Read the model definition and answer for the solid it produces. Units are mm, in the model's axes. Face numbers are marked on the shaded views. A direction names the side the tool comes from. Coordinates: 2 decimals unless noted, no trailing zeros. Write each loop counter-clockwise with the first axis right and the second up, starting at its lowest first coordinate (ties: lowest second). Pieces come first, ordered by that corner, then holes. Notation, with made-up numbers: (-19, 61.25) - (6, 61.25) arc R10 cw to (6, 67.25) - close; hole circle Ø10 at (85, 44). An arc over 180 degrees is marked (long way). Use a Markdown table: item, result.
from build123d import *

# Parameters (mm, degrees)
F0_R     = 38.1
F1_DEPTH = 76.2
F3_DEPTH = 175.006
F5_DEPTH = 304.8
F6_DEPTH = 430.022
F7_DEPTH = 172.72
F8_SIZE  = 12.7


with BuildPart() as f1:
    # F0 (on Top) → F1 (new body)
    with BuildSketch(Plane.XY):
        with BuildLine():
            Line((304.8000000003, 0), (-304.8000000003, 0))
            ThreePointArc((-304.8000000003, 0), (-358.6815367265, -22.3184632735), (-381, -76.1999999997))
            Line((-381, -76.1999999997), (-304.8000000003, -76.1999999997))
            ThreePointArc((-304.8000000003, -76.1999999997), (-228.6, -152.4), (-304.8000000003, -228.6000000003))
            Line((-304.8000000003, -228.6000000003), (-381, -228.6000000003))
            ThreePointArc((-381, -228.6000000003), (-358.6815367265, -282.4815367265), (-304.8000000003, -304.8))
            Line((-304.8000000003, -304.8), (304.8000000003, -304.8))
            ThreePointArc((304.8000000003, -304.8), (358.6815367267, -282.4815367264), (381.0000000003, -228.6))
            Line((381, -228.6000000003), (304.8000000003, -228.6000000003))
            ThreePointArc((304.8000000003, -228.6000000003), (228.6, -152.4), (304.8000000003, -76.1999999997))
            Line((304.8000000003, -76.1999999997), (381, -76.1999999997))
            ThreePointArc((381.0000000005, -76.2000000003), (358.6815367269, -22.3184632737), (304.8000000003, 0))
        make_face()
        with Locations((-177.8, -228.6)):
            Circle(F0_R, mode=Mode.SUBTRACT)
        with Locations((177.8, -228.6)):
            Circle(F0_R, mode=Mode.SUBTRACT)
        Polygon((-25.4, -114.8846255064), (-25.4, -48.2938652754), (25.4, -48.2938652754), (25.4, -114.8846255064), (101.6, -114.8846255064), (101.6, -165.6846255064), (25.4, -165.6846255064), (25.4, -241.8846255064), (-25.4, -241.8846255064), (-25.4, -165.6846255064), (-101.6, -165.6846255064), (-101.6, -114.8846255064), align=None, mode=Mode.SUBTRACT)
        with Locations((-177.7999999997, -76.2)):
            Circle(F0_R, mode=Mode.SUBTRACT)
        with Locations((177.8, -75.2889811993)):
            Circle(F0_R, mode=Mode.SUBTRACT)
        with Locations((-177.7999999997, -76.2)):
            Circle(F0_R)
        Polygon((25.4, -48.2938652754), (-25.4, -48.2938652754), (-25.4, -114.8846255064), (-101.6, -114.8846255064), (-101.6, -165.6846255064), (-25.4, -165.6846255064), (-25.4, -241.8846255064), (25.4, -241.8846255064), (25.4, -165.6846255064), (101.6, -165.6846255064), (101.6, -114.8846255064), (25.4, -114.8846255064), align=None)
        with Locations((177.8, -75.2889811993)):
            Circle(F0_R)
        with Locations((177.8, -228.6)):
            Circle(F0_R)
        with Locations((-177.8, -228.6)):
            Circle(F0_R)
    extrude(amount=-F1_DEPTH)

    # F2 (on Top) → F3 (join)
    with BuildSketch(Plane.XY):
        Polygon((25.4, -50.8), (-25.4, -50.8), (-25.4, -127), (-101.6, -127), (-101.6, -177.8), (-25.4, -177.8), (-25.4, -254), (25.4, -254), (25.4, -177.8), (101.6, -177.8), (101.6, -127), (25.4, -127), align=None)
    extrude(amount=F3_DEPTH)

    # F4 (on Front) → F5 (join)
    with BuildSketch(Plane.XZ):
        with BuildLine():
            ThreePointArc((114.3, 190.5), (-80.8223050896, 271.3223050896), (0, 76.2))
            ThreePointArc((0, 76.2), (80.8223050896, 109.6776949104), (114.3, 190.5))
        make_face()
        with BuildLine():
            ThreePointArc((76.2, 190.5), (53.8815367264, 136.6184632736), (0, 114.3))
            ThreePointArc((0, 114.3), (-53.8815367264, 244.3815367264), (76.2, 190.5))
        make_face(mode=Mode.SUBTRACT)
        with BuildLine():
            ThreePointArc((76.2, 190.5), (-53.8815367264, 244.3815367264), (0, 114.3))
            ThreePointArc((0, 114.3), (53.8815367264, 136.6184632736), (76.2, 190.5))
        make_face()
    extrude(amount=F5_DEPTH)

    # F4 (on Front) → F6 (cut)
    with BuildSketch(Plane.XZ):
        with BuildLine():
            ThreePointArc((76.2, 190.5), (-53.8815367264, 244.3815367264), (0, 114.3))
            ThreePointArc((0, 114.3), (53.8815367264, 136.6184632736), (76.2, 190.5))
        make_face()
    extrude(amount=F6_DEPTH, mode=Mode.SUBTRACT)

    # F0 (on Top) → F7 (cut)
    with BuildSketch(Plane.XY):
        with Locations((-177.7999999997, -76.2)):
            Circle(F0_R)
        with Locations((-177.8, -228.6)):
            Circle(F0_R)
        with Locations((177.8, -75.2889811993)):
            Circle(F0_R)
        with Locations((177.8, -228.6)):
            Circle(F0_R)
    extrude(amount=-F7_DEPTH, mode=Mode.SUBTRACT)

    # F8
    f8_edges = [f1.edges().sort_by_distance(p)[0] for p in [
        (139.7, -75.288981, 0),
        (139.7, -228.6, 0),
        (215.9, -228.6, -38.1),
        (139.7, -228.6, -76.2),
        (-215.9, -228.6, 0),
        (-139.7, -228.6, -38.1),
        (-215.9, -228.6, -76.2),
        (-215.9, -76.2, 0),
        (-139.7, -76.2, -38.1),
        (-215.9, -76.2, -76.2),
    ]]
    chamfer(f8_edges, length=F8_SIZE)


solid = f1.part
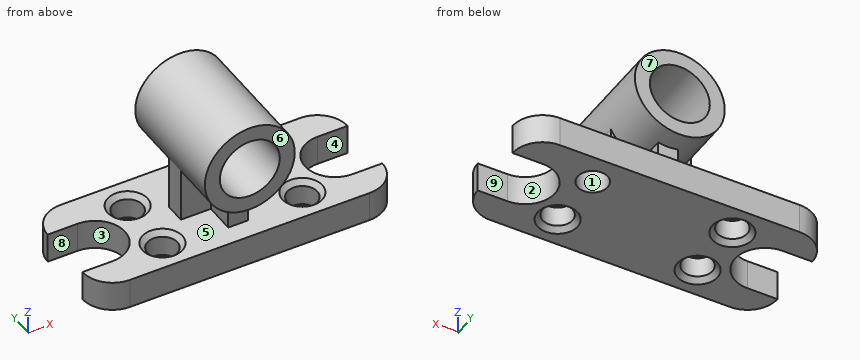
(1) A cutting plane is placed at D-D, the plane x = -294.5. Write down the section's boundary in (y, z), and give its area (3 significant figures).
Report:
| item | result |
|---|---|
| outline | (-304.8, -76.2) - (-227.9, -76.2) - (-227.9, 0) - (-304.8, 0) - close; (-76.9, -76.2) - (0, -76.2) - (0, 0) - (-76.9, 0) - close |
| area | 11,700 mm² |
(2) A cutting plane is placed at C-C, the plane z = 24.5. Write down the section's boundary in (x, y).
Report:
| item | result |
|---|---|
| outline | (-101.6, -177.8) - (-25.4, -177.8) - (-25.4, -254) - (25.4, -254) - (25.4, -177.8) - (101.6, -177.8) - (101.6, -127) - (25.4, -127) - (25.4, -50.8) - (-25.4, -50.8) - (-25.4, -127) - (-101.6, -127) - close |
(3) Straight lines are drawn through the part: L1, parallel to Y at x = 177.8, z = -61; L2, parallel to Y at x = -177.8, z = -48; L3, parallel to Z at x = 0, y = -140. For each, find the intervals that lie inside material, in ascending order.
Report:
| item | result |
|---|---|
| L1 | y = -304.8 to -266.7, -190.5 to -113.39, -37.19 to 0 |
| L2 | y = -304.8 to -266.7, -190.5 to -114.3, -38.1 to 0 |
| L3 | z = -76.2 to 114.3, 266.7 to 304.8 |
(4) A cutting plane is placed at A-A, the plane x = 177.8. Write down the section's boundary in (y, z).
Report:
| item | result |
|---|---|
| outline | (-304.8, -76.2) - (-279.4, -76.2) - (-266.7, -63.5) - (-266.7, -12.7) - (-279.4, 0) - (-304.8, 0) - close; (-190.5, -63.5) - (-177.8, -76.2) - (-113.39, -76.2) - (-113.39, -12.7) - (-126.09, 0) - (-177.8, 0) - (-190.5, -12.7) - close; (-37.19, -76.2) - (0, -76.2) - (0, 0) - (-24.49, 0) - (-37.19, -12.7) - close |
(5) A cutting plane is placed at B-B, the plane y = -153.5. Write down the section's boundary in (x, z), and give its area (3 significant figures).
Report:
| item | result |
|---|---|
| outline | (-228.61, -76.2) - (228.61, -76.2) - (228.61, 0) - (101.6, 0) - (101.6, 138.14) arc R114.3 ccw (long way) to (-101.6, 138.14) - (-101.6, 0) - (-228.61, 0) - close; hole circle Ø152.4 at (0, 190.5) |
| area | 76,700 mm² |
(6) Each of these flat-tipped pins is pushed along its axis until it touches: P1, Ø6, axis at y = -129.5, z = 79.5, coming from the -X side; P2, Ø12, axis at y = -39.5, z = 150.5, coming from the +X side; P3, Ø10, axis at x = -133, y = -261.5, coming from the +Z side. Where does it stop, or does it pass through?
Report:
| item | result |
|---|---|
| P1 | stops at x = -101.6 |
| P2 | stops at x = 109.13 |
| P3 | stops at z = 0 |
(7) The mould has two halves that part along X. Classify the marked faces 1, 2, 3 and 4: pulls with the +X half, pulls with the -X half, needs draft (parallel to the pull), parting line crosses it, or undercut.
Report:
| item | result |
|---|---|
| face 1 | undercut |
| face 2 | pulls with the +X half |
| face 3 | pulls with the -X half |
| face 4 | needs draft |
(8) For the marked faces 5, 6, 7, 8 and 9, determine the directions among +Z, -Z, +X, -X, +Y, -Y from which every point of the face is accessible in a straight line to the end or side of a thin tool.
Report:
| item | result |
|---|---|
| face 5 | none |
| face 6 | +Z, -Z, +X, -X, -Y |
| face 7 | +Z, -Z, +X, -X, +Y |
| face 8 | +Z, -Z, -X |
| face 9 | +Z, -Z, +X |
